Verification items for this drawing (mm, ordinates from the low corner). A direction names the side the tool comes from. Give positions to 0.01 mm unless a question says otherwise; leave off trailing zeros. Loops run counter-clockwise (first coordinate to the right, second up) from the corner with the lowest first, then second, coordinate; pieces in that order, holes last. Notation, with made-up numbers: (82.5, 80) -> (92.5, 80) arc R30 cw to (92.5, 119) -> close; hole circle Ø3 at (5.5, -15). An arc over 180 degrees is marked (long way). Write each question's results on one line, items separated by ' | '. Start each with the question number.
1) Sectioned sample at B-B on z = 42.5. Record the cut outline in (x, y) (3 decimals).
2) Sectioned sample at A-A on z = 35.5. Record the cut outline in (x, y) (3 decimals).
3) Scan lines: line 1 (X direction, y = 26, z = 26.5); line 2 (Z direction, x = 49, y = 36) (3 decimals). Record each from-to range of solid material in increasing order. Write a range as from..to.
4) Depth check by flat-ended pin: pin 1 (5 mm diameter, centred on x = 46, z = 5, fed in from -Y); pin 2 (2 mm diameter, centred on x = 34, z = 9, fed in from +Y); pin 3 (8 mm diameter, centred on x = 20.5, z = 9, fed in from -Y). Enter the tip coordinate at first touch or a pass-through.
5) Set-up check for the marked faces 1 and 2: record each of +Z, -Z, +X, -X, +Y, -Y from which the full face is reachable in a straight line by a thin tool's end or side.
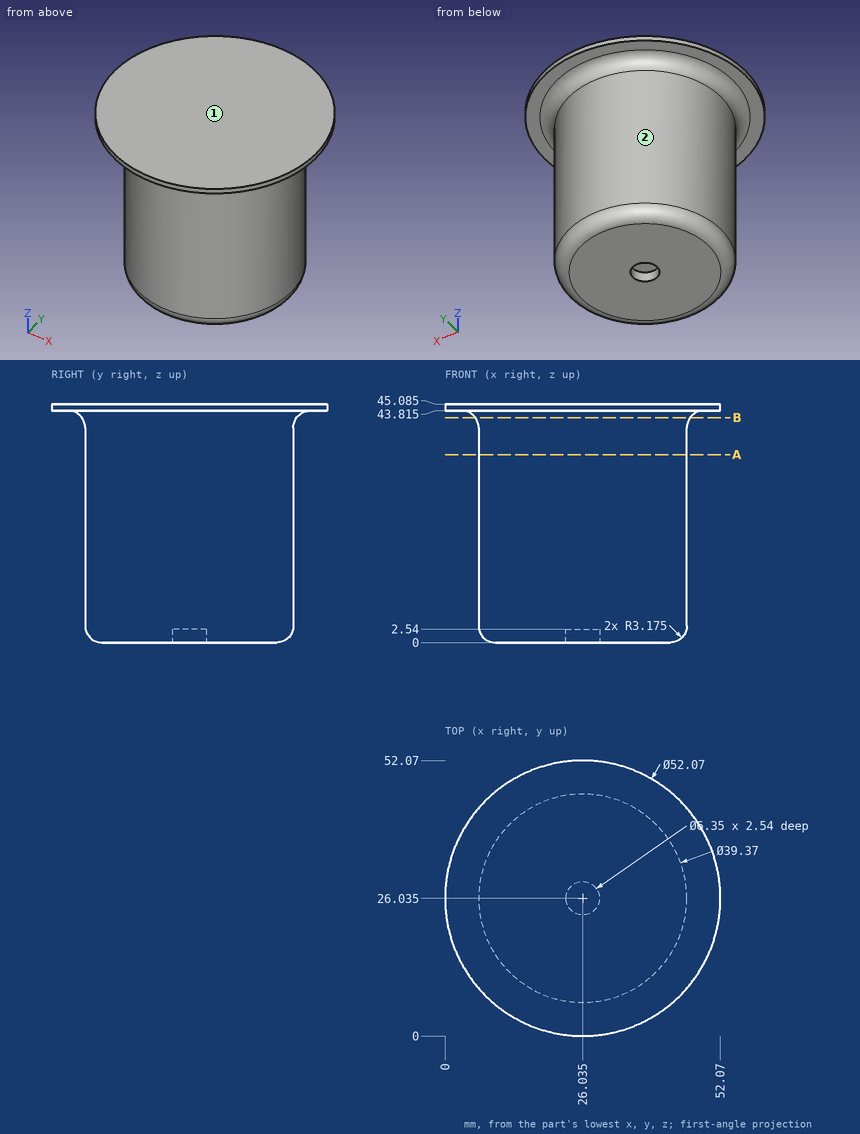
Result:
1) outline: circle Ø40.574 at (26.035, 26.035)
2) outline: circle Ø39.37 at (26.035, 26.035)
3) line 1: 6.35..45.72 | line 2: 43.815..45.085
4) pin 1: y = 16.95 | pin 2: y = 44.45 | pin 3: y = 6.41
5) face 1: +Z, +X, -X, +Y, -Y | face 2: -Z
